Geometry check sheet. Reference: the model listing, model coordinates, mm. Face numbers are marked on the shaded views. A direction names the side the tool comes from. Round coordinates to 2 decimals unless told otherwise and drop trailing zeros. Write each loop counter-clockwise with the first axis right and the second up, starting at its lowest first coordinate (ties: lowest second). Pieces come first, ordered by that corner, then holes. Notation, with made-up numbers: (1.5, -0.75) -> (28.5, -0.75) arc R26 ccw to (28.5, 15.25) -> close; hole circle Ø8 at (58.5, -36). An arc over 180 degrees is marked (long way). One line per question, with ' | ' between items.
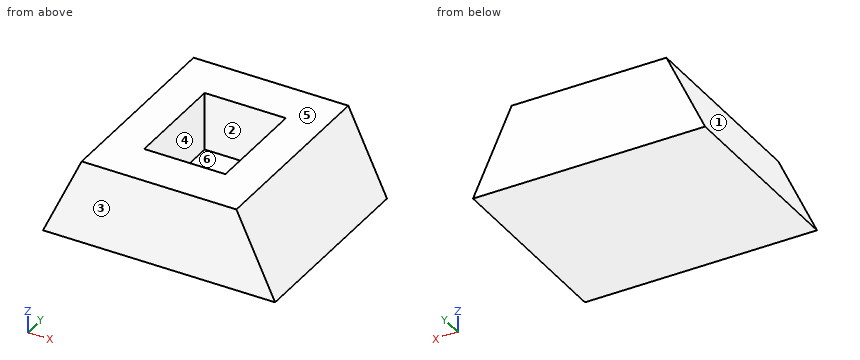
```python
from build123d import *

# Parameters (mm, degrees)
F1_DEPTH = 250
F2_W     = 105
F2_H     = 135
F3_DEPTH = 75


# Not quite as in the source:
# - a feature names something its author has since deleted; it is built from what else it names


with BuildPart() as f1:
    # F0 (on Front) → F1 (new body)
    with BuildSketch(Plane.XZ):
        Polygon((-74.1169694188, 46.7042212901), (-124.1169694188, -60.5211247353), (175.8830305812, -60.5211247353), (125.8830305812, 46.7042212901), align=None)
    extrude(amount=F1_DEPTH)

    # F2 (on face) → F3 (cut)
    with BuildSketch(Plane.XY.offset(46.7042212901)):
        with Locations((25.8830305812, -125)):
            Rectangle(F2_W, F2_H)
    extrude(amount=-F3_DEPTH, mode=Mode.SUBTRACT)


solid = f1.part
```
(1) Go/stop test with flat-tipped pins: pin 1 (8 mm diameter, centred on y = -69, z = 7, fed in from +X); pin 2 (3 mm diameter, centred on y = -66, z = 33, fed in from +X); pin 3 (1.5 mm diameter, centred on y = -147.5, z = -6, fed in from -X). Record where each tip stops, or that it passes through.
Resolved:
pin 1: stops at x = 146.26 | pin 2: stops at x = 132.97 | pin 3: stops at x = -99.04
(2) Access from +Z, -Z, +X, -X, +Y, -Y to the whole of each face (thin tool, end or side, straight path). Record for the marked faces 5 and 6.
Resolved:
face 5: +Z, +X, -X, +Y, -Y | face 6: +Z
(3) Draft check along X on the marked faces 1, 2, 3 and 4. Enter one of: +X half, -X half, draft (parallel to the pull), parting line (faces both ways), or undercut.
Resolved:
face 1: -X half | face 2: undercut | face 3: draft | face 4: undercut
(4) Sectioned sample at D-D on z = -23. Record the cut outline in (x, y), then the cut area to 3 significant figures.
Resolved:
outline: (-106.62, -250) -> (158.39, -250) -> (158.39, 0) -> (-106.62, 0) -> close; hole (-26.62, -192.5) -> (78.38, -192.5) -> (78.38, -57.5) -> (-26.62, -57.5) -> close | area: 52,100 mm2
(5) Material ranges on line 1 (Y direction, x = 4.5, z = -20); line 2 (X direction, y = -162, z = -12.5); line 3 (X direction, y = -78.5, z = 22), recorded low to high.
Resolved:
line 1: y = -250 to -192.5, -57.5 to 0 | line 2: x = -101.72 to -26.62, 78.38 to 153.49 | line 3: x = -85.64 to -26.62, 78.38 to 137.4
(6) Sectioned sample at A-A on z = 18. Record the cut outline in (x, y), then the cut area to 3 significant figures.
Resolved:
outline: (-87.5, -250) -> (139.27, -250) -> (139.27, 0) -> (-87.5, 0) -> close; hole (-26.62, -192.5) -> (78.38, -192.5) -> (78.38, -57.5) -> (-26.62, -57.5) -> close | area: 42,500 mm2
(7) Sectioned sample at C-C on x = 72.5. Record the cut outline in (y, z), then the cut area to 3 significant figures.
Resolved:
outline: (-250, -60.52) -> (0, -60.52) -> (0, 46.7) -> (-57.5, 46.7) -> (-57.5, -28.3) -> (-192.5, -28.3) -> (-192.5, 46.7) -> (-250, 46.7) -> close | area: 16,700 mm2
(8) Sectioned sample at B-B on y = -115. Record the cut outline in (x, z), then the cut area to 3 significant figures.
Resolved:
outline: (-124.12, -60.52) -> (175.88, -60.52) -> (125.88, 46.7) -> (78.38, 46.7) -> (78.38, -28.3) -> (-26.62, -28.3) -> (-26.62, 46.7) -> (-74.12, 46.7) -> close | area: 18,900 mm2
